The listing builds one solid part. Answer for the finished solid, in the listing's coordinates (mm). Face numbers are marked on the shaded views. A direction names the side the tool comes from. Coordinates: 2 decimals unless noted, no trailing zeros. Order: outer loops, then holes, each group sorted by start corner. A loop starts at its lowest first (then second) coordinate and runs counter-clockwise, first axis right, second up. Notation, with made-up numbers: (45.25, -0.5) -> (75.25, -0.5) arc R23 cw to (75.25, 19.5) -> close; hole circle Ø6 at (-26.5, -39.5). An arc over 180 degrees is marked (long way). Answer in a Markdown table with one row per item. Add a question column.
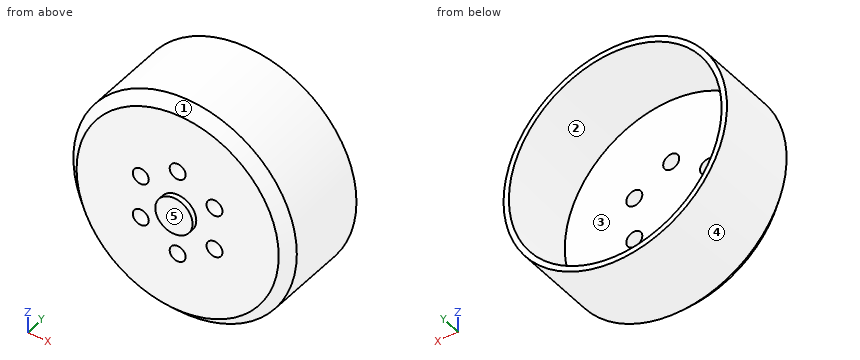
```python
from build123d import *

# Parameters (mm, degrees)
SKETCH_1_R          = 20
EXTRUDE_1_DEPTH     = 3
SKETCH_1_3_R        = 21
SKETCH_1_3_R_2      = 20
EXTRUDE_2_DEPTH     = 18
SKETCH_4_R          = 1.5
CUT_EXTRUDE_1_DEPTH = 17
SKETCH_5_R          = 3.5
EXTRUDE_3_DEPTH     = 1


with BuildPart() as part:
    # Sketch 1 → Extrude 1 (new body)
    with BuildSketch(Plane(origin=(0, 0, 0), x_dir=(1, 0, 0), z_dir=(0, 1, 0))):
        Circle(SKETCH_1_R)
    extrude(amount=EXTRUDE_1_DEPTH)

    # Sketch 1_3 → Extrude 2 (add)
    with BuildSketch(Plane(origin=(0, 0, 0), x_dir=(1, 0, 0), z_dir=(0, 1, 0))):
        Circle(SKETCH_1_3_R)
        Circle(SKETCH_1_3_R_2, mode=Mode.SUBTRACT)
    extrude(amount=EXTRUDE_2_DEPTH)

    # Sketch 3 → Cut-Revolve 1 (revolve, cut)
    with BuildSketch(Plane.XY):
        Polygon((19, 0), (21, 2), (21, 0), align=None)
    revolve(axis=Axis((0, 18, 0), (0, -1, 0)), mode=Mode.SUBTRACT)

    # Sketch 4 → Cut-Extrude 1 (cut)
    with BuildSketch(Plane.XZ):
        with Locations((0, 8)):
            Circle(SKETCH_4_R)
        with Locations((6.92820323, 4)):
            Circle(SKETCH_4_R)
        with Locations((6.92820323, -4)):
            Circle(SKETCH_4_R)
        with Locations((0, -8)):
            Circle(SKETCH_4_R)
        with Locations((-6.92820323, -4)):
            Circle(SKETCH_4_R)
        with Locations((-6.92820323, 4)):
            Circle(SKETCH_4_R)
    extrude(amount=-CUT_EXTRUDE_1_DEPTH, mode=Mode.SUBTRACT)

    # Sketch 5 → Extrude 3 (add)
    with BuildSketch(Plane.XZ):
        Circle(SKETCH_5_R)
    extrude(amount=EXTRUDE_3_DEPTH)


solid = part.part
```
Q1. A cutting plane is placed at C-C (x = 0.5). State how many separate pieces and enclosed holes the cut face has, then the cut area to 3 significant figures.
Q2. For the marked faces 1 and 2, determine the directions among +Z, -Z, +X, -X, +Y, -Y from which every point of the face is accessible in a straight line to the end or side of a thin tool.
Q3. Determine the mould class of the marked faces 3, 4 and 5 for opening direction X: +X half, -X half, draft (parallel to the pull), parting line (faces both ways), or undercut.
Q4. A cutting plane is placed at B-B (y = 9). Determine the outline of the cut face in (x, z).
Q5. A cutting plane is placed at A-A (z = 0). Determine the outline of the cut face in (x, y).
Q6. Given pin 1 (10 mm diameter, centred on x = 10, z = -4, fed in from +Y); pin 2 (2 mm diameter, centred on x = 9.5, z = 8, fed in from -Y); pin 3 (1.5 mm diameter, centred on y = 15, z = -12, fed in from -X); pin 4 (2.5 mm diameter, centred on x = 0, z = 8, fed in from +Y), each flat-ended and moving along its own axis, determine where each tip first touches the part or whether it passes through.
Q7. Straight lines are drawn through the part: line 1 (X direction, y = 2, z = -3.5); line 2 (X direction, y = 9.75, z = 0); line 3 (Z direction, x = 0, y = 1.25). For each, find the intervals that lie inside material, in ascending order.
Returned:
| question | item | result |
|---|---|---|
| 1 | separate pieces | 3 |
| 1 | enclosed holes | 0 |
| 1 | area | 142 mm² |
| 2 | face 1 | -Y |
| 2 | face 2 | +Y |
| 3 | face 3 | undercut |
| 3 | face 4 | parting line |
| 3 | face 5 | draft |
| 4 | outline | circle Ø42 at (0, 0); hole circle Ø40 at (0, 0) |
| 5 | outline | (-21, 2) -> (-19, 0) -> (-3.5, 0) -> (-3.5, -1) -> (3.5, -1) -> (3.5, 0) -> (19, 0) -> (21, 2) -> (21, 18) -> (20, 18) -> (20, 3) -> (-20, 3) -> (-20, 18) -> (-21, 18) -> close |
| 6 | pin 1 | stops at y = 3 |
| 6 | pin 2 | stops at y = 0 |
| 6 | pin 3 | stops at x = -17.73 |
| 6 | pin 4 | passes through |
| 7 | line 1 | x = -20.71 to -8.34, -5.51 to 5.51, 8.34 to 20.71 |
| 7 | line 2 | x = -21 to -20, 20 to 21 |
| 7 | line 3 | z = -20.25 to -9.5, -6.5 to 6.5, 9.5 to 20.25 |
